```python
from build123d import *

# Parameters (mm, degrees)
F0_W     = 1230
F0_H     = 630
F0_W_2   = 1200
F0_H_2   = 600
F1_DEPTH = 500
F2_W     = 40
F2_H     = 300
F3_DEPTH = 25
F4_W     = 630
F4_H     = 155
F5_DEPTH = 15


with BuildPart() as f1:
    # F0 (on Top) → F1 (new body)
    with BuildSketch(Plane.XY):
        Rectangle(F0_W, F0_H)
        Rectangle(F0_W_2, F0_H_2, mode=Mode.SUBTRACT)
    extrude(amount=F1_DEPTH)

    # F2 (on face) → F3 (cut)
    with BuildSketch(Plane(origin=(0, -300, 0), x_dir=(-1, 0, 0), z_dir=(0, 1, 0))):
        with Locations((482.5, 332)):
            Rectangle(F2_W, F2_H)
    extrude(amount=-F3_DEPTH, mode=Mode.SUBTRACT)

    # F4 (on face) → F5 (cut)
    with BuildSketch(Plane(origin=(-615, 0, 0), x_dir=(0, -1, 0), z_dir=(-1, 0, 0))):
        with Locations((0, 77.5)):
            Rectangle(F4_W, F4_H)
    extrude(amount=-F5_DEPTH, mode=Mode.SUBTRACT)


solid = f1.part
```
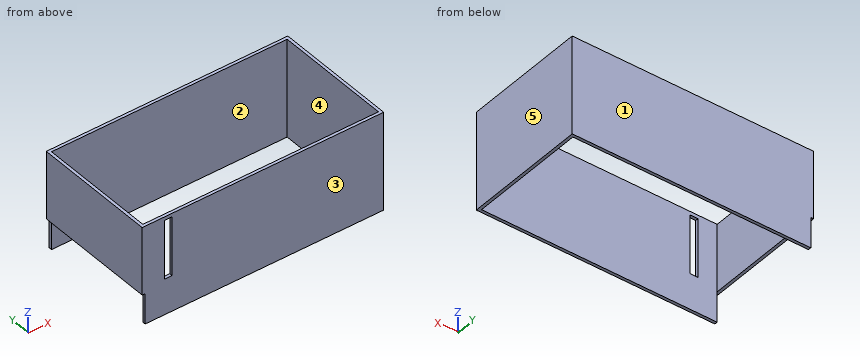
Geometry check sheet. Reference: the model listing, model coordinates, mm. Face numbers are marked on the shaded views. A direction names the side the tool comes from. Round coordinates to 2 decimals unless told otherwise and drop trailing zeros. Loops run counter-clockwise (first coordinate to the right, second up) from the corner with the lowest first, then second, coordinate; pieces in that order, holes last. Notation, with made-up numbers: M 43,-5.75 L 92,-5.75 A21 cw 92,24.25 Z; hole C -3.75,21 d5. An arc over 180 degrees is marked long. Return JSON: item names as keys, results as strings. Group by question number.
(1) Section check D-D, the plane z = 242. Enter the section's corners in (x, y), and give its area (3 significant figures).
(2) Mould release check, pull along X, two halves, no side actions. Record for the marked faces 3, 4 and 5: pulls with the +X half, pulls with the -X half, needs draft (parallel to the pull), parting line crosses it, or undercut.
(3) Scan lines: line 1 along Y through (x, z) = (196.5, 106); line 2 along X through (y, z) = (110, 397); line 3 along X through (y, z) = (287, 89). Record each from-to range of solid material in increasing order. Write a range as [from, to].
(4) Section check C-C, the plane z = 33. Enter the section's corners in (x, y), and give its area (4 significant figures).
(5) Section check B-B, the plane x = 325. Enter the section's corners in (y, z).
(6) Section check A-A, the plane y = 28.5. Enter the section's corners in (x, z).
(7) Set-up check for the marked faces 1 and 2: record each of +Z, -Z, +X, -X, +Y, -Y from which the full face is reachable in a straight line by a thin tool's end or side.
(8) Go/stop test with flat-tipped pins: pin 1 (16.5 mm diameter, centred on x = -604.5, y = 58.5, fed in from -Z); pin 2 (16.5 mm diameter, centred on y = 306, z = 71, fed in from -X). Record where each tip stops, or that it passes through.
Data:
{
 "1": {"outline": "M -615,-315 L -502.5,-315 L -502.5,-300 L -600,-300 L -600,300 L 600,300 L 600,-300 L -462.5,-300 L -462.5,-315 L 615,-315 L 615,315 L -615,315 Z", "area": "54,300 mm²"},
 "2": {"face 3": "needs draft", "face 4": "undercut", "face 5": "pulls with the +X half"},
 "3": {"line 1": "[-315, -300], [300, 315]", "line 2": "[-615, -600], [600, 615]", "line 3": "[600, 615]"},
 "4": {"outline": "M -600,-315 L 615,-315 L 615,315 L -600,315 L -600,300 L 600,300 L 600,-300 L -600,-300 Z", "area": "45,450 mm²"},
 "5": {"outline": "M -315,0 L -300,0 L -300,500 L -315,500 Z; M 300,0 L 315,0 L 315,500 L 300,500 Z"},
 "6": {"outline": "M -615,155 L -600,155 L -600,500 L -615,500 Z; M 600,0 L 615,0 L 615,500 L 600,500 Z"},
 "7": {"face 1": "+Z, -Z, +X, -X, +Y", "face 2": "+Z, -Z"},
 "8": {"pin 1": "z = 155", "pin 2": "x = -600"}
}
